The drawing under review shows one solid part. Ordinate dimensions are in mm from its lowest x, y, z. A direction names the side the tool comes from. Give positions to 0.01 mm unless a question says otherwise; leave off trailing zeros. Order: outer loops, then holes, each group sorted by start corner. A loop starts at its lowest first (then second) coordinate and runs counter-clockwise, first axis right, second up. Notation, with made-up numbers: (83.25, -5) - (97.25, -5) arc R15 cw to (97.25, 2) - close; hole circle Ø2 at (29.5, 64.5). An arc over 180 degrees is marked (long way). Use CSV: the item, a comma, the result in double quotes. Start each with the question number.
1. Machinability: for the marked faces 1, 2 and 3, which of the approach directions +Z, -Z, +X, -X, +Y, -Y give a long, thin tool a straight path to every point of the face, cutting with its end or side? Answer none if there is none.
2. Take a section at C-C, the plane z = 30. State the section outline as (x, y) points.
3. Take a section at B-B, the plane z = 6. State the section outline as (x, y) points, then the cut area to 3 significant figures.
4. Draft analysis for pull direction Z (two halves, no side actions). For the marked faces 4, 5, 6 and 7, state which applies: released by +Z, released by -Z, zero draft, split by the parting line, or undercut.
5. For pin 1 (8 mm diameter, centred on x = 7.5, y = 28, fed in from +Z); pin 2 (12 mm diameter, centred on x = 14, y = 20, fed in from -Z); pin 3 (3.5 mm diameter, centred on x = 13.5, z = 57, fed in from +Y), all flat-tipped, find the tip position at first contact; note any pin that passes through.
6. Take a section at D-D, the plane x = 18. State the section outline as (y, z) points, then the cut area to 3 significant figures.
7. To check wall thickness, follow line 1 (Z direction, x = 19, y = 22.5); line 2 (Y direction, x = 9, z = 54.35); line 3 (Z direction, x = 6, y = 3.1). State the ranges of each line that lie inside material, in increasing order. Write a range as [from, to].
8. Take a section at A-A, the plane y = 7. State the section outline as (x, z) points.
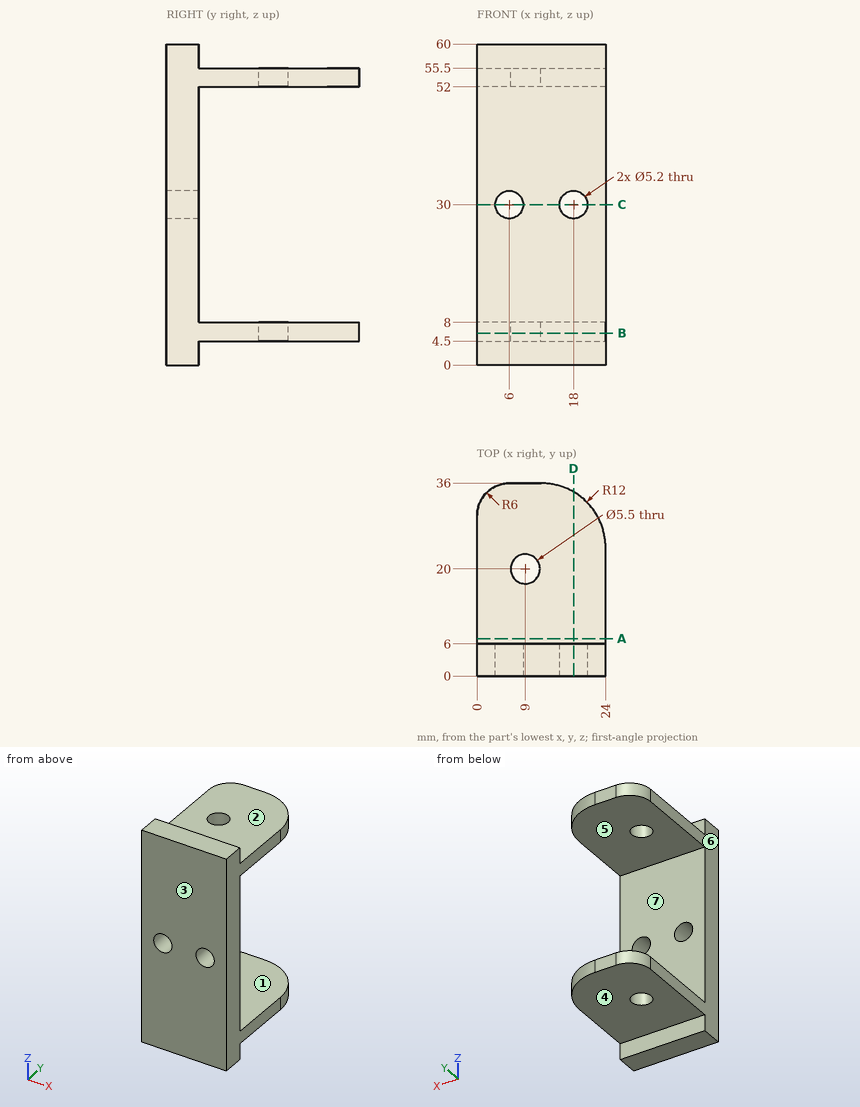
Determined:
1,face 1,"+X, -X, +Y"
1,face 2,"+Z, +X, -X, +Y"
1,face 3,"+Z, -Z, +X, -X, -Y"
2,outline,"(0, 0) - (3.4, 0) - (3.4, 6) - (0, 6) - close; (8.6, 0) - (15.4, 0) - (15.4, 6) - (8.6, 6) - close; (20.6, 0) - (24, 0) - (24, 6) - (20.6, 6) - close"
3,outline,"(0, 0) - (24, 0) - (24, 24) arc R12 ccw to (12, 36) - (6, 36) arc R6 ccw to (0, 30) - close; hole circle Ø5.5 at (9, 20)"
3,area,"802 mm²"
4,face 4,"released by -Z"
4,face 5,"undercut"
4,face 6,"zero draft"
4,face 7,"undercut"
5,pin 1,"stops at z = 55.5"
5,pin 2,"stops at z = 4.5"
5,pin 3,"stops at y = 35.99"
6,outline,"(0, 0) - (6, 0) - (6, 4.5) - (34.39, 4.5) - (34.39, 8) - (6, 8) - (6, 27.4) - (0, 27.4) - close; (0, 32.6) - (6, 32.6) - (6, 52) - (34.39, 52) - (34.39, 55.5) - (6, 55.5) - (6, 60) - (0, 60) - close"
6,area,"528 mm²"
7,line 1,"z = [4.5, 8], [52, 55.5]"
7,line 2,"y = [0, 17.25], [22.75, 36]"
7,line 3,"z = [0, 27.4], [32.6, 60]"
8,outline,"(0, 4.5) - (24, 4.5) - (24, 8) - (0, 8) - close; (0, 52) - (24, 52) - (24, 55.5) - (0, 55.5) - close"
